The listing builds one solid part. Answer for the finished solid, in the listing's coordinates (mm). A direction names the side the tool comes from. Give positions to 0.01 mm unless a question says otherwise; leave off trailing zeros. Order: outer loops, then holes, each group sorted by start corner. A loop starts at its lowest first (then second) coordinate and runs counter-clockwise, first axis right, second up.
```python
from build123d import *

# Parameters (mm, degrees)
SKETCH1_W                     = 87.5
SKETCH1_H                     = 90
SKETCH1_W_2                   = 71.5
SKETCH1_H_2                   = 71.5
BOSS_EXTRUDE1_DEPTH           = 5
M4_CLEARANCE_HOLE1_AT_2_COUNT = 2
M4_CLEARANCE_HOLE1_AT_2_PITCH = 74.042217687
SKETCH5_W                     = 10
SKETCH5_H                     = 2
BOSS_EXTRUDE2_DEPTH           = 90
SKETCH6_W                     = 87.5
SKETCH6_H                     = 7.25
CUT_EXTRUDE1_DEPTH            = 10
BOSS_EXTRUDE3_DEPTH           = 2


with BuildPart() as part:
    # Sketch1 → Boss-Extrude1 (new body)
    with BuildSketch(Plane(origin=(0, 0, 0), x_dir=(0, 0, -1), z_dir=(1, 0, 0))):
        Rectangle(SKETCH1_W, SKETCH1_H)
        with Locations((4, 0)):
            Rectangle(SKETCH1_W_2, SKETCH1_H_2, mode=Mode.SUBTRACT)
    extrude(amount=BOSS_EXTRUDE1_DEPTH)

    # Sketch4 → M4 Clearance Hole1 (revolve, cut)
    with BuildSketch(Plane(origin=(5, 40, 39.75), x_dir=(0, 0, -1), z_dir=(0, 1, 0))):
        Polygon((0, 0), (0, 9.151936393), (2.25, 7.8), (2.25, 0), align=None)
    m4_clearance_hole1 = revolve(axis=Axis((11.35, 40, 39.75), (-1, 0, 0)), mode=Mode.SUBTRACT)

    # M4 Clearance Hole1 at 2: M4 Clearance Hole1 ×2
    with Locations(*[Vector(0, 0.0337645208112264, -0.9994298160123043) * (i * M4_CLEARANCE_HOLE1_AT_2_PITCH) for i in range(1, M4_CLEARANCE_HOLE1_AT_2_COUNT)]):
        add(m4_clearance_hole1, mode=Mode.SUBTRACT)

    # Mirror1: M4 Clearance Hole1 across plane
    add(m4_clearance_hole1.mirror(Plane.ZX), mode=Mode.SUBTRACT)

    # Mirror1 copy 1 sketch → Mirror1 copy 1 (revolve, cut)
    with BuildSketch(Plane(origin=(5, -42.5, -34.25), x_dir=(0, 0, -1), z_dir=(0, -1, 0))):
        Polygon((0, 0), (0, -9.151936393), (2.25, -7.8), (2.25, 0), align=None)
    revolve(axis=Axis((11.35, -42.5, -34.25), (1, 0, 0)), mode=Mode.SUBTRACT)

    # Sketch5 → Boss-Extrude2 (add)
    with BuildSketch(Plane(origin=(0, 45, 0), x_dir=(1, 0, 0), z_dir=(0, 1, 0))):
        with Locations((10, -32.75)):
            Rectangle(SKETCH5_W, SKETCH5_H)
        Polygon((5, 41.75), (5, 39.75), (15, 28.75), (15, 30.75), align=None)
    extrude(amount=-BOSS_EXTRUDE2_DEPTH)

    # Sketch6 → Cut-Extrude1 (cut)
    with BuildSketch(Plane(origin=(5, 0, 0), x_dir=(0, 0, -1), z_dir=(1, 0, 0))):
        with Locations((0, 41.375)):
            Rectangle(SKETCH6_W, SKETCH6_H)
    cut_extrude1 = extrude(amount=CUT_EXTRUDE1_DEPTH, mode=Mode.SUBTRACT)

    # Sketch8 → Boss-Extrude3 (add)
    with BuildSketch(Plane(origin=(0, 37.75, 0), x_dir=(1, 0, 0), z_dir=(0, 1, 0))):
        Polygon((15, 28.75), (15, -31.75), (5, -31.75), (5, 39.75), align=None)
    boss_extrude3 = extrude(amount=-BOSS_EXTRUDE3_DEPTH)

    # Mirror7: Cut-Extrude1, Boss-Extrude3 across plane
    add(cut_extrude1.mirror(Plane.ZX), mode=Mode.SUBTRACT)
    add(boss_extrude3.mirror(Plane.ZX))


solid = part.part
```
1) Find section C-C (z = -8). Write down the section's boundary in (x, y), then the cut area to 4 significant figures.
Geometry says:
outline: (0, -45) - (5, -45) - (5, -37.75) - (15, -37.75) - (15, -35.75) - (0, -35.75) - close; (0, 35.75) - (15, 35.75) - (15, 37.75) - (5, 37.75) - (5, 45) - (0, 45) - close
area: 132.5 mm2
2) Find section B-B (x = 2.25). Write down the section's boundary in (y, z).
Geometry says:
outline: (-45, -43.75) - (45, -43.75) - (45, 43.75) - (-45, 43.75) - close; hole circle Ø4.5 at (-42.5, -34.25); hole circle Ø4.5 at (-40, 39.75); hole (-35.75, -39.75) - (35.75, -39.75) - (35.75, 31.75) - (-35.75, 31.75) - close; hole circle Ø4.5 at (40, 39.75); hole circle Ø4.5 at (42.5, -34.25)
3) Given P1, Ø1, axis at x = 7, y = 20.5, coming from the -Z side; P2, Ø5, axis at x = 10.5, z = 8, coming from the -Y side; P3, Ø5, axis at x = 12.5, y = 6, coming from the -Z side; P4, Ø3.5, axis at y = -40, z = 39.75, coming from the -X side, each flat-ended and moving along its own axis, determine where each tip first touches the part or whether it passes through.
Geometry says:
P1: stops at z = -40.1
P2: stops at y = -37.75
P3: stops at z = -36.25
P4: passes through
4) Find section D-D (y = -29). Write down the section's boundary in (x, z).
Geometry says:
outline: (0, -43.75) - (5, -43.75) - (5, -41.75) - (15, -30.75) - (15, -28.75) - (5, -39.75) - (0, -39.75) - close; (0, 31.75) - (15, 31.75) - (15, 33.75) - (5, 33.75) - (5, 43.75) - (0, 43.75) - close
5) A tool of negligible diameter and unlimited length cuts with its end or side. For faces 5 (the flat face through (7, 1, 31.75)), 6 (the flat face through (15, 0, -30)), 7 (the flat face through (2, -1, -39.75)), 8 (the flat face through (10, 1, 33.75)), from which of +Z, -Z, +X, -X, +Y, -Y can it reach the whole face along a straight path? Write none if from no direction.
Geometry says:
face 5: +X, -X
face 6: +Z, -Z, +X, +Y, -Y
face 7: -X
face 8: +Z, +X, +Y, -Y
6) Straight lines are drawn through the part: probe 1 along Y at (x, z) = (1.8, 39.75); probe 2 along Y at (x, z) = (2.4, -34.25); probe 3 along Y at (x, z) = (10.5, 23). For each, find the intervals that lie inside material, in ascending order.
Geometry says:
probe 1: y = -45 to -42.25, -37.75 to 37.75, 42.25 to 45
probe 2: y = -45 to -44.75, -40.25 to -35.75, 35.75 to 40.25, 44.75 to 45
probe 3: y = -37.75 to -35.75, 35.75 to 37.75
7) Find section A-A (x = 13.5). Write down the section's boundary in (y, z).
Geometry says:
outline: (-37.75, -32.4) - (37.75, -32.4) - (37.75, 33.75) - (-37.75, 33.75) - close; hole (-35.75, -30.4) - (35.75, -30.4) - (35.75, 31.75) - (-35.75, 31.75) - close
8) For a pull along Y with two mould halves and no side action, classify faces 1 (the flat face through (0, 4, 33)), 2 (the cylindrical face through (2.54, -37.77, 40.04)), 3 (the flat face through (10, -37.75, -5)), 4 (the flat face through (10, 37.75, -5)) as +Y half, -Y half, draft (parallel to the pull), parting line (faces both ways), or undercut.
Geometry says:
face 1: draft
face 2: undercut
face 3: -Y half
face 4: +Y half
